The listing builds one solid part. Answer for the finished solid, in the listing's coordinates (mm). Face numbers are marked on the shaded views. A direction names the side the tool comes from. Round coordinates to 2 decimals unless told otherwise and drop trailing zeros. Write each loop counter-clockwise with the first axis right and the second up, starting at its lowest first coordinate (ties: lowest second). Pieces come first, ordered by that corner, then holes. Notation, with made-up numbers: (17.5, -13) - (48.5, -13) arc R29 ccw to (48.5, 25) - close; hole circle Ø9 at (-36.5, 50). An arc over 180 degrees is marked (long way). Return JSON: item names as keys, results as strings. Group by question number.
(1) Section B-B, the plane z = 182 is taken. Write down the section's boundary in (x, y) (3 decimals).
(2) Determine the mould class of the marked faces 5, 6 and 7 for opening direction Y: +Y half, -Y half, draft (parallel to the pull), parting line (faces both ways), or undercut.
(3) Which of the six approach directions +Z, -Z, +X, -X, +Y, -Y give full straight-line access (tool end or side, diameter ignored) to the marked faces 1, 2, 3 and 4?
(4) Find the intervals of material crossed by line 1 along Z through (x, y) = (-120.5, 0); line 2 along Z through (x, y) = (-79.5, 0); line 3 along Z through (x, y) = (-86, -1.5), in increasing order. Write a range as [from, to].
(5) Each of these flat-tipped pins is pushed along its axis until it touches: pin 1 (10 mm diameter, centred on x = -26.5, y = 125.5, fed in from -Z); pin 2 (6.5 mm diameter, centred on y = -1, z = -136, fed in from +X); pin 3 (14 mm diameter, centred on y = -175, z = 1.5, fed in from -X). Where does it stop, or does it pass through?
```python
from build123d import *

# Parameters (mm, degrees)
BOSS_EXTRUDE3_DEPTH      = 6.35
FILLET1_R                = 6.35
CIRPATTERN5_COUNT        = 4
FILLET1_OF_CIRPATTERN5_R = 6.35
BOSS_EXTRUDE4_DEPTH      = 6.35
CIRPATTERN4_COUNT        = 4
SKETCH6_R                = 234.193665804
SKETCH6_R_2              = 215.9
CUT_EXTRUDE1_DEPTH       = 350.00288517
FILLET2_R                = 0.635
SKETCH7_R                = 60.93897947
CUT_EXTRUDE2_DEPTH       = 4.953
SKETCH8_R                = 79.670197019
CUT_EXTRUDE3_DEPTH       = 18.9484
CUT_EXTRUDE4_START       = 20.32
SKETCH11_R               = 219.71
SKETCH11_R_2             = 50.8
CUT_EXTRUDE4_DEPTH       = 20.32
CUT_EXTRUDE10_REACH      = 337.887
SKETCH20_R               = 30.226
SKETCH20_R_2             = 26.8224
CUT_EXTRUDE11_DEPTH      = 2.0066
CUT_EXTRUDE13_DEPTH      = 3.175
CIRPATTERN6_COUNT        = 8
SKETCH24_W               = 27.0002
SKETCH24_H               = 10.092146942
SKETCH25_R               = 26.6827
CUT_EXTRUDE14_DEPTH      = 20.32


with BuildPart() as part:
    # Sketch1 → Revolve2 (revolve)
    with BuildSketch(Plane.XY, mode=Mode.PRIVATE) as revolve2_sk:
        with BuildLine():
            Line((-140.081298787, 50.8), (-140.081298787, 0))
            Line((-140.081298787, 0), (-39.979898787, 0))
            Line((-39.979898787, 0), (-39.979898787, 46.736))
            Line((-39.979898787, 46.736), (-43.154898787, 46.736))
            ThreePointArc((-43.154898787, 46.736), (-47.645026847, 48.595871939), (-49.504898787, 53.086))
            Line((-49.504898787, 53.086), (-49.504898787, 219.71))
            Line((-49.504898787, 219.71), (-64.998898787, 219.71))
            Line((-64.998898787, 219.71), (-64.998898787, 63.5))
            ThreePointArc((-64.998898787, 63.5), (-68.718642666, 54.519743879), (-77.698898787, 50.8))
            Line((-77.698898787, 50.8), (-140.081298787, 50.8))
        make_face()
        with BuildLine():
            Line((-9.677698787, 219.71), (-17.678698787, 219.71))
            Line((-17.678698787, 219.71), (-17.678698787, 77.7875))
            Line((-17.678698787, 77.7875), (1.650701213, 77.7875))
            Line((1.650701213, 77.7875), (18.846501213, 77.7875))
            Line((18.846501213, 77.7875), (18.846501213, 93.599))
            ThreePointArc((18.846501213, 93.599), (18.400131948, 94.676630735), (17.322501213, 95.123))
            Line((17.322501213, 95.123), (-6.629698787, 95.123))
            ThreePointArc((-6.629698787, 95.123), (-7.707329521, 95.569369265), (-8.153698787, 96.647))
            Line((-8.153698787, 96.647), (-8.153698787, 218.186))
            ThreePointArc((-8.153698787, 218.186), (-8.600068052, 219.263630735), (-9.677698787, 219.71))
        make_face()
    revolve(revolve2_sk.sketch.rotate(Axis((-140.081298787, 0, 0), (1, 0, 0)), 180), axis=Axis((-140.081298787, 0, 0), (1, 0, 0)))

    # Sketch4 → Boss-Extrude3 (add, symmetric)
    with BuildSketch(Plane(origin=(0, 0, 0), x_dir=(1, 0, 0), z_dir=(0, -0.7071067811865488, 0.7071067811865464))):
        Polygon((-17.678698787, 219.71), (-30.378698787, 219.71), (-30.378698787, 130.302), (-36.804898787, 130.302), (-36.804898787, 219.71), (-49.504898787, 219.71), (-49.504898787, 77.7875), (-17.678698787, 77.7875), align=None)
    boss_extrude3 = extrude(amount=BOSS_EXTRUDE3_DEPTH, both=True)

    # Fillet1
    # the kernel refuses this fillet: 6.35 mm, written as the material it takes off along each edge
    with BuildSketch(Plane(origin=(-30.378698787, 87.647299742, 96.627555863), x_dir=(0, -0.7071067811865464, -0.7071067811865486), z_dir=(-1, 0, 0))) as fillet1_piece_1:
        with BuildLine():
            CenterArc((FILLET1_R, -FILLET1_R), FILLET1_R, 90, 90)
            Line((0, -FILLET1_R), (0, 0))
            Line((0, 0), (FILLET1_R, 0))
        make_face()
    extrude(amount=6.4262, mode=Mode.SUBTRACT)
    with BuildSketch(Plane(origin=(-30.378698787, 96.627555863, 87.647299742), x_dir=(0, -0.7071067811865464, -0.7071067811865486), z_dir=(-1, 0, 0))) as fillet1_piece_2:
        with BuildLine():
            CenterArc((FILLET1_R, FILLET1_R), FILLET1_R, 180, 90)
            Line((0, FILLET1_R), (0, 0))
            Line((0, 0), (FILLET1_R, 0))
        make_face()
    extrude(amount=6.4262, mode=Mode.SUBTRACT)
    with BuildSketch(Plane(origin=(-49.504898787, 59.494196802, 50.513940681), x_dir=(0, 0.707106781186547, 0.7071067811865481), z_dir=(1, 0, 0)), Plane(origin=(-49.504898787, 50.513940681, 59.494196802), x_dir=(0, 0.7071067811865492, -0.7071067811865459), z_dir=(1, 0, 0))) as fillet1_piece_3:
        with BuildLine():
            CenterArc((FILLET1_R, FILLET1_R), FILLET1_R, 180, 90)
            Line((0, FILLET1_R), (0, 0))
            Line((0, 0), (FILLET1_R, 0))
        make_face()
    extrude(amount=31.8262, mode=Mode.SUBTRACT)

    # CirPattern5: Boss-Extrude3 ×4 about axis
    cirpattern5_axis = Axis((0, 0, 0), (1, 0, 0))
    for i in range(1, CIRPATTERN5_COUNT):
        add(boss_extrude3.rotate(cirpattern5_axis, i * 360 / CIRPATTERN5_COUNT))

    # Fillet1 of CirPattern5
    # the kernel refuses this fillet: 6.35 mm, written as the material it takes off along each edge
    with BuildSketch(Plane(origin=(-30.378698787, -96.627555863, 87.647299742), x_dir=(0, 0.7071067811865509, -0.7071067811865441), z_dir=(-1, 0, 0)), Plane(origin=(-30.378698787, -87.647299742, -96.627555863), x_dir=(0, 0.7071067811865452, 0.7071067811865498), z_dir=(-1, 0, 0)), Plane(origin=(-30.378698787, 96.627555863, -87.647299742), x_dir=(0, -0.7071067811865498, 0.7071067811865454), z_dir=(-1, 0, 0))) as fillet1_of_cirpattern5_piece_1:
        with BuildLine():
            CenterArc((FILLET1_OF_CIRPATTERN5_R, -FILLET1_OF_CIRPATTERN5_R), FILLET1_OF_CIRPATTERN5_R, 90, 90)
            Line((0, -FILLET1_OF_CIRPATTERN5_R), (0, 0))
            Line((0, 0), (FILLET1_OF_CIRPATTERN5_R, 0))
        make_face()
    extrude(amount=6.4262, mode=Mode.SUBTRACT)
    with BuildSketch(Plane(origin=(-30.378698787, -87.647299742, 96.627555863), x_dir=(0, 0.7071067811865509, -0.7071067811865441), z_dir=(-1, 0, 0)), Plane(origin=(-30.378698787, -96.627555863, -87.647299742), x_dir=(0, 0.7071067811865441, 0.7071067811865509), z_dir=(-1, 0, 0)), Plane(origin=(-30.378698787, 87.647299742, -96.627555863), x_dir=(0, -0.7071067811865509, 0.7071067811865441), z_dir=(-1, 0, 0))) as fillet1_of_cirpattern5_piece_2:
        with BuildLine():
            CenterArc((FILLET1_OF_CIRPATTERN5_R, FILLET1_OF_CIRPATTERN5_R), FILLET1_OF_CIRPATTERN5_R, 180, 90)
            Line((0, FILLET1_OF_CIRPATTERN5_R), (0, 0))
            Line((0, 0), (FILLET1_OF_CIRPATTERN5_R, 0))
        make_face()
    extrude(amount=6.4262, mode=Mode.SUBTRACT)
    with BuildSketch(Plane(origin=(-49.504898787, -50.513940681, 59.494196802), x_dir=(0, -0.7071067811865475, 0.7071067811865475), z_dir=(1, 0, 0)), Plane(origin=(-49.504898787, -59.494196802, 50.513940681), x_dir=(0, 0.7071067811865464, 0.7071067811865486), z_dir=(1, 0, 0)), Plane(origin=(-49.504898787, -59.494196802, -50.513940681), x_dir=(0, -0.7071067811865481, -0.707106781186547), z_dir=(1, 0, 0)), Plane(origin=(-49.504898787, -50.513940681, -59.494196802), x_dir=(0, -0.7071067811865486, 0.7071067811865464), z_dir=(1, 0, 0)), Plane(origin=(-49.504898787, 50.513940681, -59.494196802), x_dir=(0, 0.7071067811865476, -0.7071067811865476), z_dir=(1, 0, 0)), Plane(origin=(-49.504898787, 59.494196802, -50.513940681), x_dir=(0, -0.7071067811865459, -0.7071067811865492), z_dir=(1, 0, 0))) as fillet1_of_cirpattern5_piece_3:
        with BuildLine():
            CenterArc((FILLET1_OF_CIRPATTERN5_R, FILLET1_OF_CIRPATTERN5_R), FILLET1_OF_CIRPATTERN5_R, 180, 90)
            Line((0, FILLET1_OF_CIRPATTERN5_R), (0, 0))
            Line((0, 0), (FILLET1_OF_CIRPATTERN5_R, 0))
        make_face()
    extrude(amount=31.8262, mode=Mode.SUBTRACT)

    # Sketch5 → Boss-Extrude4 (add, symmetric)
    with BuildSketch(Plane(origin=(0, 0, 0), x_dir=(-1, 0, 0), z_dir=(0, 0, -1))):
        Polygon((49.504898787, 219.71), (49.504898787, 73.66), (36.804898787, 86.36), (36.804898787, 219.71), align=None)
        Polygon((17.678698787, 77.7875), (17.678698787, 219.71), (30.378698787, 219.71), (30.378698787, 90.4875), align=None)
    boss_extrude4 = extrude(amount=BOSS_EXTRUDE4_DEPTH, both=True)

    # CirPattern4: Boss-Extrude4 ×4 about axis
    cirpattern4_axis = Axis((0, 0, 0), (1, 0, 0))
    for i in range(1, CIRPATTERN4_COUNT):
        add(boss_extrude4.rotate(cirpattern4_axis, i * 360 / CIRPATTERN4_COUNT))

    # Sketch6 → Cut-Extrude1 (cut, through all)
    with BuildSketch(Plane.ZY.offset(140.081298787)):
        Circle(SKETCH6_R)
        with Locations(Location((0, 0, 0), (0, 0, 270))):
            Circle(SKETCH6_R_2, mode=Mode.SUBTRACT)
    extrude(amount=-CUT_EXTRUDE1_DEPTH, mode=Mode.SUBTRACT)

    # Fillet2
    fillet2_edges = [part.edges().sort_by_distance(p)[0] for p in [
        (-39.979898787, 46.736, 0),
    ]]
    fillet(fillet2_edges, radius=FILLET2_R)

    # Sketch7 → Cut-Extrude2 (cut)
    with BuildSketch(Plane(origin=(-39.979898787, 0, 0), x_dir=(0, 0, -1), z_dir=(1, 0, 0))):
        Circle(SKETCH7_R)
    extrude(amount=-CUT_EXTRUDE2_DEPTH, mode=Mode.SUBTRACT)

    # Sketch8 → Cut-Extrude3 (cut)
    with BuildSketch(Plane.ZY.offset(140.081298787)):
        Circle(SKETCH8_R)
    extrude(amount=-CUT_EXTRUDE3_DEPTH, mode=Mode.SUBTRACT)

    # Sketch11 → Cut-Extrude4 (cut)
    with BuildSketch(Plane.ZY.offset(64.998898787).offset(CUT_EXTRUDE4_START)):
        Circle(SKETCH11_R)
        with Locations(Location((0, 0, 0), (0, 0, 270))):
            Circle(SKETCH11_R_2, mode=Mode.SUBTRACT)
    extrude(amount=-CUT_EXTRUDE4_DEPTH, mode=Mode.SUBTRACT)

    # Sketch12 → Cut-Revolve1 (revolve, cut)
    with BuildSketch(Plane(origin=(0, 0, 0), x_dir=(1, 0, 0), z_dir=(0, 1, 0)), mode=Mode.PRIVATE) as cut_revolve1_sk:
        with BuildLine():
            Line((-121.132898787, 31.75), (-80.111898787, 31.75))
            ThreePointArc((-80.111898787, 31.75), (-76.957987839, 32.588616713), (-74.637123327, 34.882961973))
            Line((-74.637123327, 34.882961973), (-65.874123327, 49.795890249))
            ThreePointArc((-65.874123327, 49.795890249), (-65.613530636, 50.287482958), (-65.396970658, 50.8))
            Line((-65.396970658, 50.8), (-121.132898787, 50.8))
            Line((-121.132898787, 50.8), (-121.132898787, 31.75))
        make_face()
    revolve(cut_revolve1_sk.sketch.rotate(Axis((-60.172898787, 0, 0), (-1, 0, 0)), 270), axis=Axis((-60.172898787, 0, 0), (-1, 0, 0)), mode=Mode.SUBTRACT)

    # Sketch18 → Cut-Extrude10 (cut, up to next)
    with BuildSketch(Plane.ZY.offset(121.132898787), mode=Mode.PRIVATE) as cut_extrude10_sk1:
        with BuildLine():
            Line((-14.359429538, -21.094621628), (-21.094621628, -14.359429538))
            Line((-21.094621628, -14.359429538), (-17.575856913, -10.840664823))
            ThreePointArc((-17.575856913, -10.840664823), (14.601896453, 14.601896453), (-10.840664823, -17.575856913))
            Line((-10.840664823, -17.575856913), (-14.359429538, -21.094621628))
        make_face()
    cut_extrude10_tool1 = extrude(cut_extrude10_sk1.sketch, amount=-CUT_EXTRUDE10_REACH, mode=Mode.PRIVATE) & part.part
    add(cut_extrude10_tool1.solids().sort_by_distance((-121.132899, -0.51024, -0.51024))[0], mode=Mode.SUBTRACT)

    # Sketch20 → Cut-Extrude11 (cut)
    with BuildSketch(Plane.ZY.offset(121.132898787)):
        with Locations(Location((0, 0, 0), (0, 0, 270))):
            Circle(SKETCH20_R)
        with Locations(Location((0, 0, 0), (0, 0, 270))):
            Circle(SKETCH20_R_2, mode=Mode.SUBTRACT)
    extrude(amount=-CUT_EXTRUDE11_DEPTH, mode=Mode.SUBTRACT)

    # Sketch22 → Cut-Extrude13 (cut)
    with BuildSketch(Plane.ZY.offset(64.998898787)):
        with BuildLine():
            Line((50.92871008, 64.399094261), (145.78051919, 159.250903372))
            ThreePointArc((145.78051919, 159.250903372), (82.621353048, 199.465591069), (9.525, 215.689787368))
            Line((9.525, 215.689787368), (9.525, 84.123223233))
            ThreePointArc((9.525, 84.123223233), (24.00104092, 61.192302667), (50.92871008, 64.399094261))
        make_face()
    cut_extrude13 = extrude(amount=-CUT_EXTRUDE13_DEPTH, mode=Mode.SUBTRACT)

    # CirPattern6: Cut-Extrude13 ×8 about axis
    cirpattern6_axis = Axis((0, 0, 0), (1, 0, 0))
    for i in range(1, CIRPATTERN6_COUNT):
        add(cut_extrude13.rotate(cirpattern6_axis, i * 360 / CIRPATTERN6_COUNT), mode=Mode.SUBTRACT)

    # Sketch24 → Cut-Revolve2 (revolve, cut)
    with BuildSketch(Plane(origin=(0, 0, 0), x_dir=(1, 0, 0), z_dir=(0, 1, 0)), mode=Mode.PRIVATE) as cut_revolve2_sk:
        with Locations((5.346401213, 95.533573471)):
            Rectangle(SKETCH24_W, SKETCH24_H)
    revolve(cut_revolve2_sk.sketch.rotate(Axis((-154.951085714, 0, 0), (1, 0, 0)), 271.68541304), axis=Axis((-154.951085714, 0, 0), (1, 0, 0)), mode=Mode.SUBTRACT)

    # Sketch25 → Cut-Extrude14 (cut)
    with BuildSketch(Plane(origin=(-44.932898787, 0, 0), x_dir=(0, 0, -1), z_dir=(1, 0, 0))):
        with Locations(Location((0, 0, 0), (0, 0, 90))):
            Circle(SKETCH25_R)
    extrude(amount=-CUT_EXTRUDE14_DEPTH, mode=Mode.SUBTRACT)


solid = part.part
```
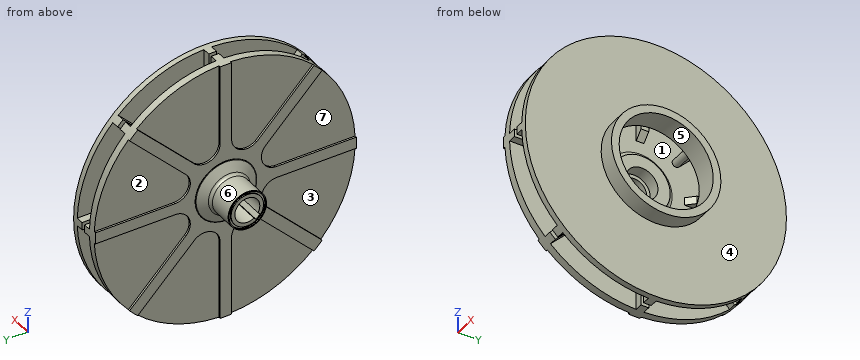
Working result:
{
 "1": {"outline": "(-64.999, -9.525) - (-61.824, -9.525) - (-61.824, -116.141) - (-49.505, -116.141) - (-49.505, -6.35) - (-36.805, -6.35) - (-36.805, 6.35) - (-49.505, 6.35) - (-49.505, 116.141) - (-61.824, 116.141) - (-61.824, 9.525) - (-64.999, 9.525) - close; (-30.379, -6.35) - (-17.679, -6.35) - (-17.679, -116.141) - (-8.154, -116.141) - (-8.154, 116.141) - (-17.679, 116.141) - (-17.679, 6.35) - (-30.379, 6.35) - close"},
 "2": {"face 5": "undercut", "face 6": "parting line", "face 7": "draft"},
 "3": {"face 1": "none", "face 2": "-X, +Y", "face 3": "-X, -Y", "face 4": "+X"},
 "4": {"line 1": "z = [-31.75, -30.23], [-26.82, -20.65], [20.65, 26.82], [30.23, 31.75]", "line 2": "z = [-31.78, -20.65], [20.65, 31.78]", "line 3": "z = [-31.71, -20.6], [20.6, 31.71]"},
 "5": {"pin 1": "stops at z = -139.48", "pin 2": "stops at x = -8.15", "pin 3": "stops at x = -65"}
}
